Geometry check sheet. Reference: the model listing, model coordinates, mm. A direction names the side the tool comes from. Round coordinates to 2 decimals unless told otherwise and drop trailing zeros. Write each loop counter-clockwise with the first axis right and the second up, starting at its lowest first coordinate (ties: lowest second). Pieces come first, ordered by that corner, then holes. Notation, with made-up numbers: (-12.75, 46.25) - (45.25, 46.25) arc R23 ccw to (45.25, 82.25) - close; hole circle Ø6 at (68.25, 9). An arc over 180 degrees is marked (long way). Return JSON: item names as keys, results as strings.
Autodesk Inventor part; units mm, degrees
ref_plane "YZ Plane" through (0, 0, 0) normal (1, 0, 0) x (0, 1, 0)
ref_plane "XZ Plane" through (0, 0, 0) normal (0, 1, 0) x (-1, 0, 0)
ref_plane "XY Plane" through (0, 0, 0) normal (0, 0, 1) x (1, 0, 0)
sketch "Sketch1" plane through (0, 0, 0) normal (0, 1, 0) x (-1, 0, 0)
  line L0 (100, -50) -> (-100, -50)
  line L1 (-100, -50) -> (-100, 50)
  line L2 (-100, 50) -> (100, 50)
  line L3 (100, 50) -> (100, -50)
  line L4 (100, -50) -> (-100, 50) construction
  line L5 (-100, -50) -> (100, 50) construction
  line L6 (-40, -30) -> (-80, -30)
  line L7 (-50, -50) -> (-70, -50)
  line L8 (-40, -30) -> (-50, -50)
  line L9 (-80, -30) -> (-70, -50)
  line L10 (80, -30) -> (40, -30)
  line L11 (70, -50) -> (50, -50)
  line L12 (80, -30) -> (70, -50)
  line L13 (40, -30) -> (50, -50)
  line L14 (-100, -10) -> (-100, 10)
  line L15 (-80, -20) -> (-80, 20)
  line L16 (-80, -20) -> (-100, -10)
  line L17 (-80, 20) -> (-100, 10)
  line L18 (100, -50) -> (-100, -50)
  line L19 (-100, -50) -> (-130, -50)
  line L20 (-130, -50) -> (-130, 50)
  line L21 (-130, 50) -> (-100, 50)
  line L22 (-100, 50) -> (-100, -50)
  line L23 (-120, -20) -> (-120, 20)
  line L24 (-120, -20) -> (-100, -10)
  line L25 (-120, 20) -> (-100, 10)
  point P0 (0, 0)
  point P1 (-100, 10)
  point P2 (-100, -10)
  point P3 (-70, -50)
  point P4 (-50, -50)
  point P5 (70, -50)
  point P6 (0, 0)
  point P7 (0, 0)
  point P8 (-100, -50)
  dimension "d72" = 200
  dimension "d73" = 100
  dimension "d78" = 20
  dimension "d79" = 40
  dimension "d80" = 20
  dimension "d81" = 10
  dimension "d82" = 20
  dimension "d83" = 40
  dimension "d84" = 20
  dimension "d85" = 10
  dimension "d86" = 120
  dimension "d87" = 30
  dimension "d88" = 0
  dimension "d89" = 0
  dimension "d90" = 40
  dimension "d91" = 20
  dimension "d92" = 20
  dimension "d93" = 10
  dimension "d94" = 40
  dimension "d95" = 0
  dimension "d122" = 30
extrude "Extrusion24" add sketch "Sketch1" along normal blind 12 contours L1 L25 L23 L24 L19 L20 L21 | L1 L24 L23 L25
extrude "Extrusion25" cut sketch "Sketch1" along normal blind 6 contours L1 L24 L23 L25
fillet "Fillet11" radius 2 2 edges at (120, 3, 20) (120, 3, -20)
fillet "Fillet12" radius 6 2 edges at (130, 0, 0) (130, 12, 0)
properties part number "Test2_3DPrint"
(1) Section check B-B, the plane x = 107. Enter the section's corners in (y, z), plus the area to 3 significant figures.
Response values:
{"outline": "(0, -50) - (12, -50) - (12, 50) - (0, 50) - (0, 13.5) - (6, 13.5) - (6, -13.5) - (0, -13.5) - close", "area": "1,040 mm^2"}
(2) Release check for a two-part mould opening along Z. For faces 1 (the face through (115, 6, 50)), 2 (the face through (128.196, 1.711, 0.7)), 3 (the face through (108.673, 2.958, 14.336)) record: pulls with the +Z half, pulls with the -Z half, needs draft (parallel to the pull), parting line crosses it, or undercut.
Response values:
{"face 1": "pulls with the +Z half", "face 2": "needs draft", "face 3": "undercut"}
(3) Section check D-D, the plane x = 118.75. Enter the section's corners in (y, z).
Response values:
{"outline": "(0, -50) - (12, -50) - (12, 50) - (0, 50) - (0, 18.62) - (6, 18.62) - (6, -18.62) - (0, -18.62) - close"}
(4) Access from +Z, -Z, +X, -X, +Y, -Y to the whole of each face (thin tool, end or side, straight path). Record for faces 4 (the face through (119.076, 3.042, -18.45)), 5 (the face through (115, 6, -50)).
Response values:
{"face 4": "-Y", "face 5": "-Z, +X, -X, +Y, -Y"}
(5) Section check C-C, the plane y = 1.75. Enter the section's corners in (x, z).
Response values:
{"outline": "(100, -50) - (128.24, -50) - (128.24, 50) - (100, 50) - (100, 10) - (117.11, 18.55) arc R2 cw to (120, 16.76) - (120, -16.76) arc R2 cw to (117.11, -18.55) - (100, -10) - close"}
(6) Gauge pin test, flat end, axial feed: pin 1 (5 mm diameter, centred on y = 3, z = -3, fed in from -X). Record the tip position at first contact, or that the pin passes through.
Response values:
{"pin 1": "stops at x = 120"}
(7) Material ranges on line 1 along Y through (x, z) = (113, 2); line 2 along Z through (x, y) = (112.25, 5.5) (3 decimals); line 3 along Z through (x, y) = (113.25, 5.25) (3 decimals), recorded low to high. Write a range as [from, to].
Response values:
{"line 1": "y = [6, 12]", "line 2": "z = [-50, -16.125], [16.125, 50]", "line 3": "z = [-50, -16.625], [16.625, 50]"}
